The drawing under review shows one solid part. Ordinate dimensions are in mm from its lowest x, y, z. A direction names the side the tool comes from. Coordinates: 2 decimals unless noted, no trailing zeros. Order: outer loops, then holes, each group sorted by start corner. A loop starts at its lowest first (then second) coordinate and runs counter-clockwise, first axis right, second up. Notation, with made-up numbers: M -27,39.5 L -19,39.5 A20 cw -19,50.5 Z; hole C -1,67 d7. An arc over 180 degrees is marked long. Answer as a JSON object with one key per item and string values.
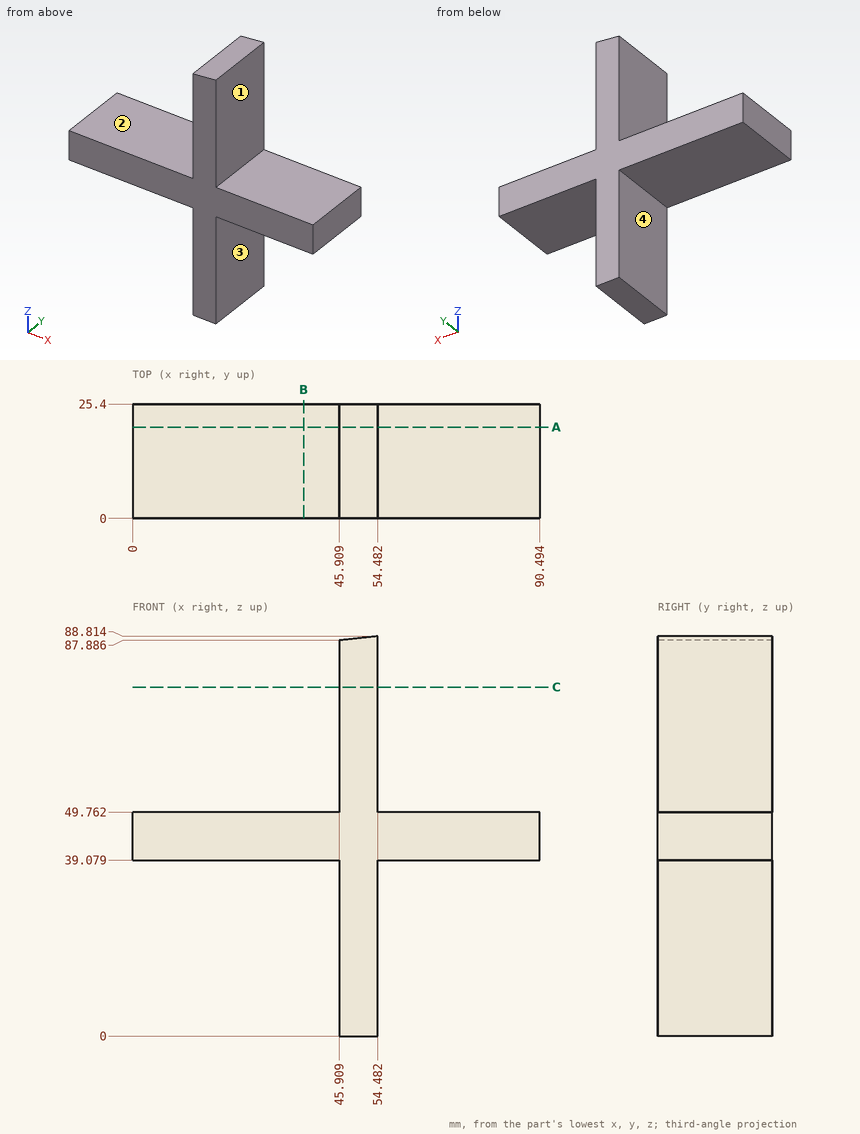
1) To check wall thickness, follow L1, parallel to X at y = 24, z = 76; L2, parallel to Z at x = 29.5, y = 14. State the ranges of each line that lie inside material, in increasing order.
Taken from the geometry:
{"L1": "x = 45.91 to 54.48", "L2": "z = 39.08 to 49.76"}
2) Tool access review of the marked faces 1, 2, 3 and 4: name each direction out of +Z, -Z, +X, -X, +Y, -Y from which nothing blocks a thin tool from reaching the whole face with its end or side.
Taken from the geometry:
{"face 1": "+Z, +X, +Y, -Y", "face 2": "+Z, -X, +Y, -Y", "face 3": "-Z, +X, +Y, -Y", "face 4": "-Z, -X, +Y, -Y"}
3) Add section A-A (y = 20.25). State the section outline as (x, z) points (1 decimal).
Taken from the geometry:
{"outline": "M 0,39.1 L 45.9,39.1 L 45.9,0 L 54.5,0 L 54.5,39.1 L 90.5,39.1 L 90.5,49.8 L 54.5,49.8 L 54.5,88.8 L 45.9,87.9 L 45.9,49.8 L 0,49.8 Z"}
4) Add section B-B (x = 38). State the section outline as (y, z) points, and give its area (3 significant figures).
Taken from the geometry:
{"outline": "M 0,39.08 L 25.4,39.08 L 25.4,49.76 L 0,49.76 Z", "area": "271 mm2"}
5) Add section C-C (z = 77.5). State the section outline as (x, y) points, and give its area (3 significant figures).
Taken from the geometry:
{"outline": "M 45.91,0 L 54.48,0 L 54.48,25.4 L 45.91,25.4 Z", "area": "218 mm2"}
6) Insertion check: pin 1 Ø12.5 at (x, y) = (80, 18.5) entering from +Z; pin 2 Ø1 at (x, y) = (73.5, 20.5) entering from -Z; pin 3 Ø8 at (y, z) = (15.5, 76) entering from +X. Each pin has a flat end and moves straight along its axis. Give the tip position at first contact, or say it passes through.
Taken from the geometry:
{"pin 1": "stops at z = 49.76", "pin 2": "stops at z = 39.08", "pin 3": "stops at x = 54.48"}
